Verification items for the finished model (mm, model axes). Face numbers are marked on the shaded views. A direction names the side the tool comes from. Round coordinates to 2 decimals unless told otherwise and drop trailing zeros. Loops run counter-clockwise (first coordinate to the right, second up) from the corner with the lowest first, then second, coordinate; pieces in that order, holes last. Notation, with made-up numbers: (83.5, 89.25) - (122.5, 89.25) arc R25 cw to (122.5, 120.25) - close; hole circle Ø3 at (86, -30.5). An arc over 180 degrees is marked (long way). Use CSV: the item, a comma, the result in double quotes.
```python
from build123d import *

# Parameters (mm, degrees)
BOSS_EXTRUDE1_DEPTH = 7
SKETCH2_R           = 4.1
CUT_EXTRUDE1_DEPTH  = 30.722213915
CHAMFER1_SIZE       = 0.5
CHAMFER2_SIZE       = 0.3


with BuildPart() as part:
    # Sketch1 → Boss-Extrude1 (new, symmetric)
    with BuildSketch(Plane.XY):
        Polygon((-21.1, 14), (-21.1, 4), (21.1, 4), (21.1, 14), (27.1, 14), (27.1, 0), (-27.1, 0), (-27.1, 14), align=None)
    extrude(amount=BOSS_EXTRUDE1_DEPTH, both=True)

    # Sketch2 → Cut-Extrude1 (cut, through all)
    with BuildSketch(Plane(origin=(0, 4, 0), x_dir=(1, 0, 0), z_dir=(0, 1, 0))):
        with Locations(Location((0, 0, 0), (0, 0, 270))):
            Circle(SKETCH2_R)
    extrude(amount=-CUT_EXTRUDE1_DEPTH, mode=Mode.SUBTRACT)

    # Chamfer1
    chamfer1_edges = [part.edges().sort_by_distance(p)[0] for p in [
        (27.1, 7, -7),
        (0, 0, -7),
        (-27.1, 7, -7),
        (-24.1, 14, -7),
        (0, 0, 7),
        (-21.1, 14, 0),
        (21.1, 14, 0),
        (27.1, 14, 0),
        (27.1, 0, 0),
        (-27.1, 0, 0),
        (-27.1, 14, 0),
        (27.1, 7, 7),
        (24.1, 14, 7),
        (21.1, 9, 7),
        (0, 4, 7),
        (-21.1, 9, 7),
        (-24.1, 14, 7),
        (-21.1, 9, -7),
        (-27.1, 7, 7),
        (0, 4, -7),
        (21.1, 9, -7),
        (24.1, 14, -7),
    ]]
    chamfer(chamfer1_edges, length=CHAMFER1_SIZE)

    # Chamfer2
    chamfer2_edges = [part.edges().sort_by_distance(p)[0] for p in [
        (0, 0, -4.1),
        (0, 4, -4.1),
    ]]
    chamfer(chamfer2_edges, length=CHAMFER2_SIZE)


solid = part.part
```
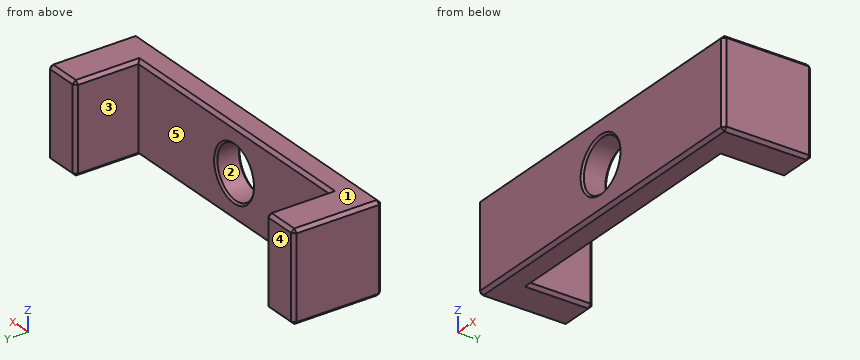
1) Access from +Z, -Z, +X, -X, +Y, -Y to the whole of each face (thin tool, end or side, straight path). Record for the marked faces 4 and 5.
Returned:
face 4,"+Z, -Z, +X, -X, +Y"
face 5,"+Z, -Z, +Y"
2) Cross-section at C-C, the plane x = 0. Record the cut outline in (y, z).
Returned:
outline,"(0, -6.5) - (0.5, -7) - (3.5, -7) - (4, -6.5) - (4, -4.4) - (3.7, -4.1) - (0.3, -4.1) - (0, -4.4) - close; (0, 4.4) - (0.3, 4.1) - (3.7, 4.1) - (4, 4.4) - (4, 6.5) - (3.5, 7) - (0.5, 7) - (0, 6.5) - close"
3) Cross-section at D-D, the plane y = 2.75. Record the cut outline in (x, z).
Returned:
outline,"(-27.1, -6.5) - (-26.6, -7) - (26.6, -7) - (27.1, -6.5) - (27.1, 6.5) - (26.6, 7) - (-26.6, 7) - (-27.1, 6.5) - close; hole circle Ø8.2 at (0, 0)"
4) Cross-section at B-B, the plane z = 0. Record the cut outline in (x, y), then the cut area to 3 significant figures.
Returned:
outline,"(-27.1, 0.5) - (-26.6, 0) - (-4.4, 0) - (-4.1, 0.3) - (-4.1, 3.7) - (-4.4, 4) - (-21.1, 4) - (-21.1, 13.5) - (-21.6, 14) - (-26.6, 14) - (-27.1, 13.5) - close; (4.1, 0.3) - (4.4, 0) - (26.6, 0) - (27.1, 0.5) - (27.1, 13.5) - (26.6, 14) - (21.6, 14) - (21.1, 13.5) - (21.1, 4) - (4.4, 4) - (4.1, 3.7) - close"
area,"303 mm²"
5) Gauge pin test, flat end, axial feed: pin 1 Ø6 at (x, z) = (-12, -2.5) entering from +Y. Record the tip position at first contact, or that the pin passes through.
Returned:
pin 1,"stops at y = 4"
6) Cross-section at A-A, the plane y = 11.25. Record the cut outline in (x, z).
Returned:
outline,"(-27.1, -6.5) - (-26.6, -7) - (-21.6, -7) - (-21.1, -6.5) - (-21.1, 6.5) - (-21.6, 7) - (-26.6, 7) - (-27.1, 6.5) - close; (21.1, -6.5) - (21.6, -7) - (26.6, -7) - (27.1, -6.5) - (27.1, 6.5) - (26.6, 7) - (21.6, 7) - (21.1, 6.5) - close"
7) Thickness scan on probe 1 along X at (y, z) = (2.5, 0); probe 2 along X at (y, z) = (7.5, 3); probe 3 along Y at (x, z) = (-9, 0). Record the ranges inside material, lowest first. Write a range as [from, to].
Returned:
probe 1,"x = [-27.1, -4.1], [4.1, 27.1]"
probe 2,"x = [-27.1, -21.1], [21.1, 27.1]"
probe 3,"y = [0, 4]"
8) Mould release check, pull along Z, two halves, no side actions. Record for the marked faces 1, 2 and 3: +Z half, -Z half, draft (parallel to the pull), parting line (faces both ways), or undercut.
Returned:
face 1,"+Z half"
face 2,"undercut"
face 3,"draft"
